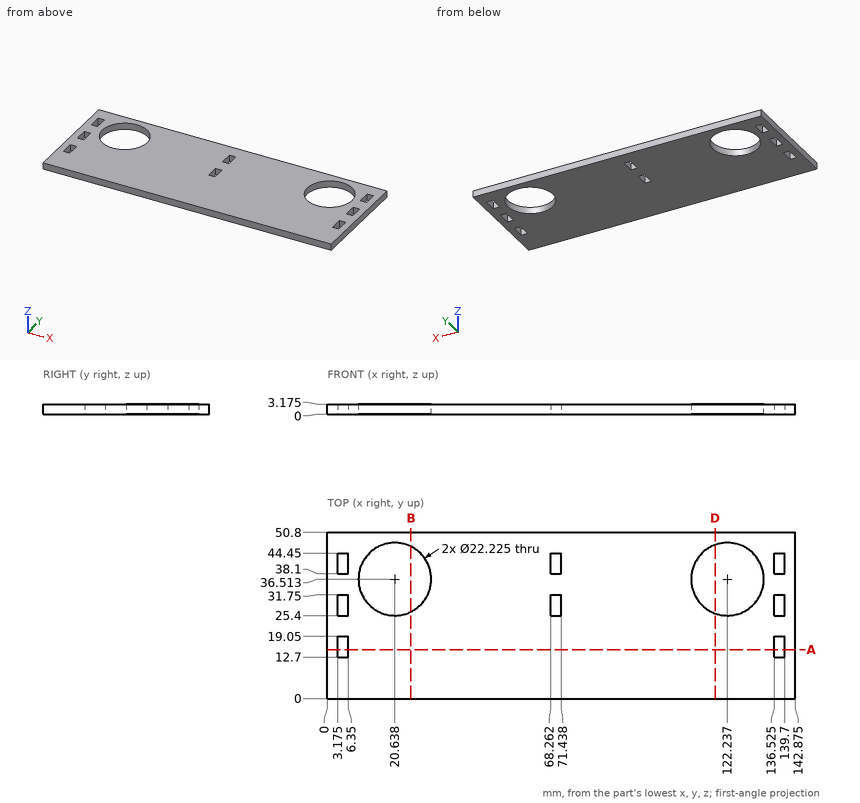
Input: dimensioned drawing with shaded views. Units: mm. Origin: part minimum x, y, z. Coordinates: 2 decimals unless noted, no trailing zeros. Order: outer loops, then holes, each group sorted by start corner. A loop starts at its lowest first (then second) coordinate and runs counter-clockwise, first axis right, second up. Notation, with made-up numbers: (-40, -7) -> (17, -7) arc R22 cw to (17, 15) -> close; hole circle Ø5 at (55, 70). An arc over 180 degrees is marked (long way). Answer in a Markdown table with one row per item.
Item 1: Section D-D on x = 118.5. Output: boundary loops of the cut face in (y, z) (1 decimal).
Return value:
| item | result |
|---|---|
| outline | (0, 0) -> (26, 0) -> (26, 3.2) -> (0, 3.2) -> close; (47, 0) -> (50.8, 0) -> (50.8, 3.2) -> (47, 3.2) -> close |
Item 2: Ray query, L1, parallel to X at y = 37, z = 2.2 (1 decimal); L2, parallel to Y at x = 68.5, z = 0.3; L3, parallel to Y at x = 121, z = 2.4 (1 decimal). Return the intervals inside material, ascending.
Return value:
| item | result |
|---|---|
| L1 | x = 0 to 9.5, 31.7 to 111.1, 133.3 to 142.9 |
| L2 | y = 0 to 25.4, 31.75 to 38.1, 44.45 to 50.8 |
| L3 | y = 0 to 25.5, 47.6 to 50.8 |
Item 3: Contact query for a flat-ended pin moving along its axis: P1, Ø13.5, axis at x = 20.64, y = 36.51, coming from the +Z side. Output: stop coordinate, or through.
Return value:
| item | result |
|---|---|
| P1 | passes through |
Item 4: Section A-A on y = 15. State how many separate pieces and enclosed holes the cut face has.
Return value:
| item | result |
|---|---|
| separate pieces | 3 |
| enclosed holes | 0 |
Item 5: Section B-B on x = 25.5. Output: boundary loops of the cut face in (y, z) (1 decimal).
Return value:
| item | result |
|---|---|
| outline | (0, 0) -> (26.5, 0) -> (26.5, 3.2) -> (0, 3.2) -> close; (46.5, 0) -> (50.8, 0) -> (50.8, 3.2) -> (46.5, 3.2) -> close |
